Build history of the part. All positions in model axes, mm. A direction names the side the tool comes from. Round coordinates to 2 decimals unless told otherwise and drop trailing zeros. Loops run counter-clockwise (first coordinate to the right, second up) from the corner with the lowest first, then second, coordinate; pieces in that order, holes last. Notation, with made-up numbers: M 37,9 L 87,9 A14 cw 87,30 Z; hole C -34.75,61.5 d5. An arc over 180 degrees is marked long. One line per item, written item: value.
```python
from build123d import *

# Parameters (mm, degrees)
F0_W     = 215
F0_H     = 16
F1_DEPTH = 8
F2_R     = 2.5
F3_DEPTH = 7
F4_R     = 3
F5_R     = 1
F6_R     = 1.5
F7_W     = 210
F7_H     = 5
F8_DEPTH = 5.5


with BuildPart() as f1:
    # F0 (on Top) → F1 (new body)
    with BuildSketch(Plane.XY):
        with Locations((-7.5, 0)):
            Rectangle(F0_W, F0_H)
    extrude(amount=F1_DEPTH)

    # F2 (on face) → F3 (join)
    with BuildSketch(Plane(origin=(0, 0, 0), x_dir=(1, 0, 0), z_dir=(0, 0, -1))):
        with Locations((-77.5, 0)):
            Circle(F2_R)
        with Locations((82.5, 0)):
            Circle(F2_R)
    extrude(amount=F3_DEPTH)

    # F4
    f4_edges = [f1.edges().sort_by_distance(p)[0] for p in [
        (-115, -8, 4),
        (-115, 8, 4),
    ]]
    fillet(f4_edges, radius=F4_R)

    # F5
    f5_edges = [f1.edges().sort_by_distance(p)[0] for p in [
        (-80, 0, -7),
        (80, 0, -7),
    ]]
    fillet(f5_edges, radius=F5_R)

    # F6
    f6_edges = [f1.edges().sort_by_distance(p)[0] for p in [
        (-6, -8, 8),
    ]]
    fillet(f6_edges, radius=F6_R)

    # F7 (on face) → F8 (cut)
    with BuildSketch(Plane.XY.offset(8)):
        with Locations((-5, 0)):
            Rectangle(F7_W, F7_H)
    extrude(amount=-F8_DEPTH, mode=Mode.SUBTRACT)


solid = f1.part
```
Item 1: Drop flat-ended pins along their axis: P1, Ø8, axis at x = 10.5, y = -0.5, coming from the -Z side; P2, Ø4, axis at y = 1, z = 4, coming from the +X side; P3, Ø4, axis at y = -3.5, z = -5, coming from the -X side; P4, Ø2, axis at y = 2.5, z = -5, coming from the +X side. Give the stop position or say it passes through.
Check values:
P1: stops at z = 0
P2: stops at x = 100
P3: stops at x = -79.5
P4: stops at x = 84.5
Item 2: Slice it at B-B, the plane z = -4. Give the cut face in (x, y), and give its area (3 significant figures).
Check values:
outline: C -77.5,0 d5; C 82.5,0 d5
area: 39.3 mm2
Item 3: Pull direction Y, two halves, no side cores. Call faces 4 (the face through (-6, -2.5, 5)), 5 (the face through (-7, 8, 3)), 6 (the face through (-9, 0, 0)): pulls with the +Y half, pulls with the -Y half, needs draft (parallel to the pull), parting line crosses it, or undercut.
Check values:
face 4: undercut
face 5: pulls with the +Y half
face 6: needs draft
Item 4: Slice it at A-A, the plane x = -72.5. Give the cut face in (y, z).
Check values:
outline: M -8,0 L 8,0 L 8,6.5 A1.5 ccw 6.5,8 L 2.5,8 L 2.5,2.5 L -2.5,2.5 L -2.5,8 L -6.5,8 A1.5 ccw -8,6.5 Z
Item 5: Which spindle directions (+Z, -Z, +X, -X, +Y, -Y) get a long thin tool onto all of the face, cutting with end or side? Do faces 1 (the face through (100, 0, 2)), 2 (the face through (-80, 0, -3)), 3 (the face through (-110, 0, 5)). Say none if no direction does.
Check values:
face 1: +Z, -Z, +X, +Y, -Y
face 2: -Z
face 3: +Z, +X
Item 6: Wall check: line 1 along Y through (x, z) = (-41, 6.5); line 2 along Z through (x, y) = (-36, 0.5); line 3 along Z through (x, y) = (-26.5, -4.5). Give the ranges that are in metal, low to high.
Check values:
line 1: y = -8 to -2.5, 2.5 to 8
line 2: z = 0 to 2.5
line 3: z = 0 to 8
